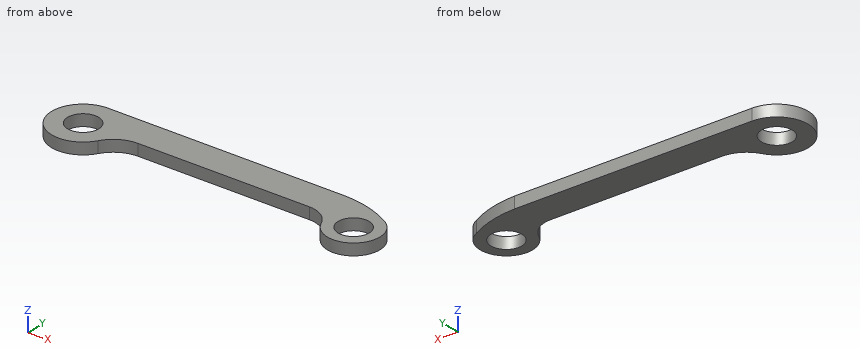
from build123d import *

# Parameters (mm, degrees)
SKETCH2_R           = 19.2
SKETCH2_R_2         = 9.472
SKETCH2_R_3         = 16
BOSS_EXTRUDE1_DEPTH = 7


with BuildPart() as part:
    # Sketch2 → Boss-Extrude1 (new body)
    # profile 1 of 3: a face of its own
    with BuildSketch(Plane.XY):
        with BuildLine():
            Line((144.339154619, 19.2), (0, 19.2))
            ThreePointArc((0, 19.2), (13.576450199, 13.576450199), (19.2, 0))
            ThreePointArc((19.2, 0), (18.545775865, -4.969325666), (16.627687753, -9.6))
            ThreePointArc((16.627687753, -9.6), (23.655375505, -2.572312247), (33.255375505, 0))
            Line((33.255375505, 0), (137.316262944, 0))
            ThreePointArc((137.316262944, 0), (146.079689306, -2.613351487), (151.980376503, -9.5997052))
            ThreePointArc((151.980376503, -9.5997052), (155.441326908, 8.223773716), (173.328738352, 11.337467698))
            ThreePointArc((173.328738352, 11.337467698), (159.301290335, 16.991856013), (144.339154619, 19.2))
        make_face()
    # profile 2 of 3: a face of its own
    with BuildSketch(Plane.XY):
        Circle(SKETCH2_R)
        Circle(SKETCH2_R_2, mode=Mode.SUBTRACT)
    # profile 3 of 3: a face of its own
    with BuildSketch(Plane.XY):
        with Locations((166.644490062, -3.199410399)):
            Circle(SKETCH2_R_3)
        with Locations((166.644490062, -3.199410399)):
            Circle(SKETCH2_R_2, mode=Mode.SUBTRACT)
    extrude(amount=BOSS_EXTRUDE1_DEPTH)


solid = part.part
Check sheet for the modelled part. Datum: model origin and axes. Units: mm. Give positions to 0.01 mm unless a question says otherwise; leave off trailing zeros. Loops run counter-clockwise (first coordinate to the right, second up) from the corner with the lowest first, then second, coordinate; pieces in that order, holes last. Notation, with made-up numbers: M 8,-14.75 L 18,-14.75 A12 ccw 18,2.25 Z; hole C -29.5,-8.75 d5. An arc over 180 degrees is marked long. Return JSON: item names as keys, results as strings. Group by question number.
1. Go/stop test with flat-tipped pins: pin 1 (1.5 mm diameter, centred on y = 15, z = 5, fed in from -X); pin 2 (4 mm diameter, centred on y = -12.5, z = 3, fed in from -X); pin 3 (8 mm diameter, centred on x = 14, y = 8, fed in from -Z); pin 4 (2 mm diameter, centred on x = 78, z = 4, fed in from -Y). Record where each tip stops, or that it passes through.
2. Cross-section at C-C on y = -15. Record the boundary of the cut face in (x, z) (3 decimals), plus the area to 3 significant figures.
3. Cross-section at D-D on x = 47. Record the boundary of the cut face in (y, z).
4. Thickness scan on L1, parallel to X at y = -1.5, z = 5; L2, parallel to X at y = 1.5, z = 5.75; L3, parallel to Y at x = 0.5, z = 6. Record the ranges inside material, lowest first.
5. Cross-section at A-A on y = 2. Record the boundary of the cut face in (x, z), plus the area to 3 significant figures.
6. Cross-section at B-B on z = 5.25. Record the boundary of the cut face in (x, y), plus the area to 3 significant figures.
Return value:
{
 "1": {"pin 1": "x = -12.87", "pin 2": "x = -16.07", "pin 3": "z = 0", "pin 4": "y = 0"},
 "2": {"outline": "M -11.985,0 L 11.985,0 L 11.985,7 L -11.985,7 Z; M 155.84,0 L 177.449,0 L 177.449,7 L 155.84,7 Z", "area": "319 mm^2"},
 "3": {"outline": "M 0,0 L 19.2,0 L 19.2,7 L 0,7 Z"},
 "4": {"L1": "-19.14 to -9.35, 9.35 to 25.82, 144.08 to 157.33, 175.96 to 182.55", "L2": "-19.14 to -9.35, 9.35 to 158.42, 174.87 to 181.94", "L3": "-19.19 to -9.46, 9.46 to 19.2"},
 "5": {"outline": "M -19.1,0 L -9.26,0 L -9.26,7 L -19.1,7 Z; M 9.26,0 L 158.73,0 L 158.73,7 L 9.26,7 Z; M 174.56,0 L 181.78,0 L 181.78,7 L 174.56,7 Z", "area": "1,170 mm^2"},
 "6": {"outline": "M 0,19.2 A19.2 ccw long 16.63,-9.6 A19.2 cw 33.26,0 L 137.32,0 A16 cw 151.98,-9.6 A16 ccw long 173.33,11.34 A64.06 ccw 144.34,19.2 Z; hole C 0,0 d18.94; hole C 166.64,-3.2 d18.94", "area": "4,190 mm^2"}
}
